Design review of the part built by this model. Coordinates are the model's own, in mm. Face numbers are marked on the shaded views. A direction names the side the tool comes from. Give positions to 0.01 mm unless a question says otherwise; leave off trailing zeros. Loops run counter-clockwise (first coordinate to the right, second up) from the corner with the lowest first, then second, coordinate; pieces in that order, holes last. Notation, with made-up numbers: (4.25, 67) - (13.25, 67) arc R7 cw to (13.25, 73) - close; hole circle Ø3 at (-14.5, 14). An arc over 180 degrees is marked (long way). Write each question's results on one line, items separated by ' | '.
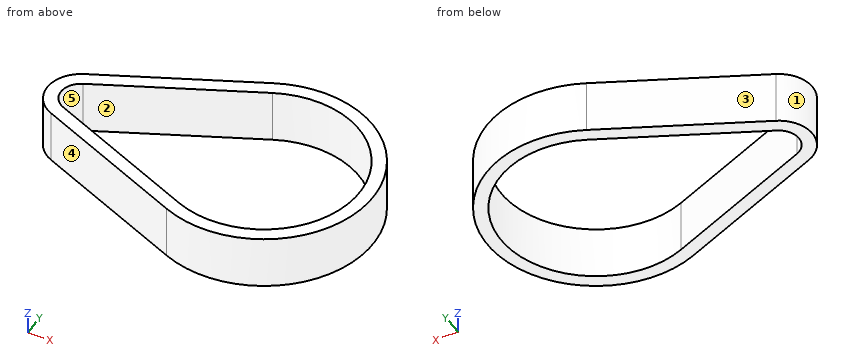
Autodesk Inventor part; units mm, degrees
ref_plane "YZ Plane" through (0, 0, 0) normal (1, 0, 0) x (0, 1, 0)
ref_plane "XZ Plane" through (0, 0, 0) normal (0, 1, 0) x (-1, 0, 0)
ref_plane "XY Plane" through (0, 0, 0) normal (0, 0, 1) x (1, 0, 0)
sketch "Sketch1" plane through (0, 0, 0) normal (0, 0, 1) x (1, 0, 0)
  circle A0 centre (0, 0) radius 7.26 construction
  line L0 (0, 0) -> (51.5, 0) construction
  arc A1 (-2.3048, 5.1684) -> (-2.3048, -5.1684) centre (0, 0) ccw
  arc A2 (9.469, 0) -> (4.6289, 8.2604) centre (0, 0) ccw construction
  circle A3 centre (51.5, 0) radius 28.265 construction
  arc A4 (40.6525, -24.3249) -> (40.6525, 24.3249) centre (51.5, 0) ccw
  arc A5 (21.056, 0) -> (27.1842, -18.3188) centre (51.5, 0) ccw construction
  line L1 (-3.8565, 8.6481) -> (39.1007, 27.8046)
  line L2 (-3.8565, -8.6481) -> (39.1007, -27.8046)
  line L3 (-2.3048, 5.1684) -> (40.6525, 24.3249)
  line L4 (-2.3048, -5.1684) -> (40.6525, -24.3249)
  arc A6 (24.866, 0) -> (40.6525, -24.3249) centre (51.5, 0) ccw construction
  arc A7 (40.6525, 24.3249) -> (24.866, 0) centre (51.5, 0) ccw construction
  arc A8 (5.659, 0) -> (-2.3048, 5.1684) centre (0, 0) ccw construction
  arc A9 (-2.3048, -5.1684) -> (5.659, 0) centre (0, 0) ccw construction
  arc A10 (4.6289, -8.2604) -> (9.469, 0) centre (0, 0) ccw construction
  arc A11 (4.6289, 8.2604) -> (-3.8565, 8.6481) centre (0, 0) ccw construction
  arc A12 (27.1842, 18.3188) -> (21.056, 0) centre (51.5, 0) ccw construction
  arc A13 (27.1842, -18.3188) -> (39.1007, -27.8046) centre (51.5, 0) ccw construction
  arc A14 (-3.8565, 8.6481) -> (-3.8565, -8.6481) centre (0, 0) ccw
  arc A15 (-3.8565, -8.6481) -> (4.6289, -8.2604) centre (0, 0) ccw construction
  arc A16 (39.1007, 27.8046) -> (27.1842, 18.3188) centre (51.5, 0) ccw construction
  arc A17 (39.1007, -27.8046) -> (39.1007, 27.8046) centre (51.5, 0) ccw
  dimension "d0" = 14.52
  dimension "d1" = 51.5
  dimension "d4" = 56.53
  dimension "d10" = 3.81
  dimension "d12" = 3.81
  dimension "d13" = 1.601
  dimension "d14" = 1.631
extrude "Extrusion1" add sketch "Sketch1" along normal blind 15
properties part number "Belt" material "Rubber, Silicone"
(1) Tool access review of the marked faces 1 and 2: name each direction out of +Z, -Z, +X, -X, +Y, -Y from which nothing blocks a thin tool from reaching the whole face with its end or side.
Answers below:
face 1: +Z, -Z, -X | face 2: +Z, -Z
(2) Take a section at A-A on y = 0. Give the boundary of the cut face in (x, z).
Answers below:
outline: (-9.47, 0) - (-5.66, 0) - (-5.66, 15) - (-9.47, 15) - close; (78.13, 0) - (81.94, 0) - (81.94, 15) - (78.13, 15) - close
(3) Wall thickness on line 1 along Y through (x, z) = (51.5, 6); line 2 along X through (y, z) = (0, 10.5); line 3 along Y through (x, z) = (23, 6.75): over which ranges is each line inside the solid? List them lowest first. Write a range as from..to.
Answers below:
line 1: -30.44..-26.63, 26.63..30.44 | line 2: -9.47..-5.66, 78.13..81.94 | line 3: -20.62..-16.45, 16.45..20.62
(4) Insertion check: P1, Ø1.5, axis at y = -13, z = 8.5, coming from the -X side; P2, Ø2, axis at y = -19, z = 11.5, coming from the +X side; P3, Ø8, axis at x = 37.5, z = 3.5, coming from the +Y side. Each pin has a flat end and moves straight along its axis. Give the tip position at first contact, or say it passes through.
Answers below:
P1: x = 4.22 | P2: x = 76.05 | P3: y = 28.75
(5) Take a section at B-B on z = 10. Give the boundary of the cut face in (x, y).
Answers below:
outline: (-3.86, -8.65) - (39.1, -27.8) arc R30.44 ccw (long way) to (39.1, 27.8) - (-3.86, 8.65) arc R9.47 ccw to start; hole (-2.3, -5.17) - (40.65, -24.32) arc R26.63 ccw (long way) to (40.65, 24.32) - (-2.3, 5.17) arc R5.66 ccw to start
(6) Draft analysis for pull direction Y (two halves, no side actions). For the marked faces 3, 4 and 5, state which applies: pulls with the +Y half, pulls with the -Y half, needs draft (parallel to the pull), parting line crosses it, or undercut.
Answers below:
face 3: pulls with the +Y half | face 4: pulls with the -Y half | face 5: undercut
(7) Take a section at C-C on x = 51.5. Give the boundary of the cut face in (y, z).
Answers below:
outline: (-30.44, 0) - (-26.63, 0) - (-26.63, 15) - (-30.44, 15) - close; (26.63, 0) - (30.44, 0) - (30.44, 15) - (26.63, 15) - close
